CAD build for the part. Positions are in the model's coordinates, mm. Coordinates: 2 decimals unless noted, no trailing zeros. Loops run counter-clockwise (first coordinate to the right, second up) from the corner with the lowest first, then second, coordinate; pieces in that order, holes last. Notation, with made-up numbers: (25, 62) -> (33, 62) arc R25 cw to (33, 75) -> close; hole circle Ø8 at (-18, -34.75). An arc over 180 degrees is marked (long way). Return JSON: item names as keys, results as strings. Group by question number.
(1) Saw through at A-A on x = 0. Write the cut outline in (y, z), then the cut area to 3 significant figures.
(2) Saw through at D-D on x = -0.85. Write the cut outline in (y, z).
(3) Mould opens along X. For faces 1 (the face through (-3, 0, 10)), 2 (the face through (-0.07, -0.04, 14.5)), 3 (the face through (0, 0, 0)), 4 (the face through (3, 0, 10)) say: pulls with the +X half, pulls with the -X half, needs draft (parallel to the pull), parting line crosses it, or undercut.
(4) Saw through at C-C on y = 2.3. Write the cut outline in (x, z), then the cut area to 3 significant figures.
(5) Probe L1, parallel to Z at x = -0.1, y = -0.1; L2, parallel to Y at x = 0.4, z = 8; L3, parallel to Z at x = 0.75, y = -1.35. List the from-to ranges inside material, lowest first.
(6) Saw through at B-B on z = 13. Write the cut outline in (x, y).
```python
from build123d import *

# Parameters (mm, degrees)
SKETCH_1_W               = 6
SKETCH_1_H               = 6
EXTRUDE_1_DEPTH          = 21
CUT_EXTRUDE_1_DEPTH      = 21
CUT_EXTRUDE_1_DEPTH_BACK = 21
SKETCH_3_R               = 1.5
CUT_EXTRUDE_2_DEPTH      = 21
CUT_EXTRUDE_2_DEPTH_BACK = 21
SKETCH_4_R               = 1.5
FILLET_1_R               = 0.5


with BuildPart() as part:
    # 草图1 → 凸台-拉伸1 (new body)
    with BuildSketch(Plane.XY):
        Rectangle(SKETCH_1_W, SKETCH_1_H)
    extrude(amount=EXTRUDE_1_DEPTH)

    # 草图3 → 切除-拉伸1 (cut, two sides: drawn at the far end of the back side and taken through both)
    with BuildSketch(Plane(origin=(0, 0, 0), x_dir=(1, 0, 0), z_dir=(0, 1, 0)).offset(-CUT_EXTRUDE_1_DEPTH_BACK)):
        with Locations(Location((0, -3, 0), (0, 0, 90))):
            Circle(SKETCH_3_R)
        with Locations(Location((0, -13, 0), (0, 0, 90))):
            Circle(SKETCH_3_R)
    extrude(amount=CUT_EXTRUDE_1_DEPTH + CUT_EXTRUDE_1_DEPTH_BACK, mode=Mode.SUBTRACT)

    # 草图4 → 切除-拉伸2 (cut, two sides: drawn at the far end of the back side and taken through both)
    with BuildSketch(Plane(origin=(0, 0, 0), x_dir=(0, 0, -1), z_dir=(1, 0, 0)).offset(-CUT_EXTRUDE_2_DEPTH_BACK)):
        with Locations(Location((-18, 0, 0), (0, 0, 180))):
            Circle(SKETCH_4_R)
        with Locations(Location((-8, 0, 0), (0, 0, 180))):
            Circle(SKETCH_4_R)
    extrude(amount=CUT_EXTRUDE_2_DEPTH + CUT_EXTRUDE_2_DEPTH_BACK, mode=Mode.SUBTRACT)

    # 圆角1
    fillet_1_edges = [part.edges().sort_by_distance(p)[0] for p in [
        (3, -3, 10.5),
        (-3, -3, 10.5),
        (-3, 3, 10.5),
        (3, 3, 10.5),
    ]]
    fillet(fillet_1_edges, radius=FILLET_1_R)


solid = part.part
```
Geometry results:
{
 "1": {"outline": "(-3, 0) -> (3, 0) -> (3, 1.5) -> (-3, 1.5) -> close; (-3, 4.5) -> (3, 4.5) -> (3, 11.5) -> (-3, 11.5) -> close; (-3, 14.5) -> (3, 14.5) -> (3, 21) -> (-3, 21) -> close; hole circle Ø3 at (0, 8); hole circle Ø3 at (0, 18)", "area": "75.9 mm²"},
 "2": {"outline": "(-3, 0) -> (3, 0) -> (3, 1.76) -> (-3, 1.76) -> close; (-3, 4.24) -> (3, 4.24) -> (3, 11.76) -> (-3, 11.76) -> close; (-3, 14.24) -> (3, 14.24) -> (3, 21) -> (-3, 21) -> close; hole circle Ø3 at (0, 8); hole circle Ø3 at (0, 18)"},
 "3": {"face 1": "pulls with the -X half", "face 2": "undercut", "face 3": "needs draft", "face 4": "pulls with the +X half"},
 "4": {"outline": "(-3, 0) -> (3, 0) -> (3, 21) -> (-3, 21) -> close; hole circle Ø3 at (0, 3); hole circle Ø3 at (0, 13)", "area": "112 mm²"},
 "5": {"L1": "0 to 1.5, 4.5 to 6.5, 9.5 to 11.5, 14.5 to 16.5, 19.5 to 21", "L2": "-3 to -1.5, 1.5 to 3", "L3": "0 to 1.7, 4.3 to 7.35, 8.65 to 11.7, 14.3 to 17.35, 18.65 to 21"},
 "6": {"outline": "(-3, -2.5) arc R0.5 ccw to (-2.5, -3) -> (-1.5, -3) -> (-1.5, 3) -> (-2.5, 3) arc R0.5 ccw to (-3, 2.5) -> close; (1.5, -3) -> (2.5, -3) arc R0.5 ccw to (3, -2.5) -> (3, 2.5) arc R0.5 ccw to (2.5, 3) -> (1.5, 3) -> close"}
}
